Input: part model. Units: mm. Frame: model coordinates. A direction names the side the tool comes from. Coordinates: 2 decimals unless noted, no trailing zeros. Order: outer loops, then holes, each group sorted by start corner. A loop starts at its lowest first (then second) coordinate and runs counter-clockwise, first axis right, second up. Notation, with made-up numbers: (-27, -31) - (7, -31) arc R33 cw to (7, -3) - close; hole circle Ø5 at (3.25, 78.25). An arc over 180 degrees is marked (long way). One line per question, with ' | ' between items.
from build123d import *

# Parameters (mm, degrees)
SKETCH1_R           = 3
SKETCH1_R_2         = 2
BOSS_EXTRUDE1_DEPTH = 5


with BuildPart() as part:
    # Sketch1 → Boss-Extrude1 (new body)
    with BuildSketch(Plane(origin=(0, 0, 0), x_dir=(0, 0, -1), z_dir=(1, 0, 0))):
        Polygon((-32.401546808, -7.5), (3.598453192, -7.5), (6.598453192, -4.5), (24.598453192, -4.5), (27.598453192, -7.5), (63.598453192, -7.5), (54.938199155, 7.5), (51.938199155, 7.5), (45.876021328, 18), (51.938199155, 28.5), (54.938199155, 28.5), (63.598453192, 43.5), (27.598453192, 43.5), (24.598453192, 40.5), (6.598453192, 40.5), (3.598453192, 43.5), (-32.401546808, 43.5), (-23.74129277, 28.5), (-20.74129277, 28.5), (-14.679114943, 18), (-20.74129277, 7.5), (-23.74129277, 7.5), align=None)
        Circle(SKETCH1_R, mode=Mode.SUBTRACT)
        with Locations((38.848942605, 0)):
            Circle(SKETCH1_R, mode=Mode.SUBTRACT)
        with Locations((31.196906385, 36)):
            Circle(SKETCH1_R, mode=Mode.SUBTRACT)
        with Locations((-7.65203622, 36)):
            Circle(SKETCH1_R, mode=Mode.SUBTRACT)
        with Locations((15.598453192, 18)):
            Circle(SKETCH1_R_2, mode=Mode.SUBTRACT)
        with Locations((-2.401546808, 18)):
            Circle(SKETCH1_R_2, mode=Mode.SUBTRACT)
        with Locations((33.598453192, 18)):
            Circle(SKETCH1_R_2, mode=Mode.SUBTRACT)
    extrude(amount=BOSS_EXTRUDE1_DEPTH)


solid = part.part
Item 1: Section D-D on z = -22.5. Return the cut outline in (x, y).
Data:
outline: (0, -4.5) - (5, -4.5) - (5, 40.5) - (0, 40.5) - close
Item 2: Section C-C on z = -40. Return the cut outline in (x, y).
Data:
outline: (0, -7.5) - (5, -7.5) - (5, -2.77) - (0, -2.77) - close; (0, 2.77) - (5, 2.77) - (5, 43.5) - (0, 43.5) - close
Item 3: Ray query, line 1 (Y direction, x = 1.5, z = 0); line 2 (Z direction, x = 4.1, y = 35); line 3 (Z direction, x = 3.55, y = -5). Return the intervals inside material, ascending.
Data:
line 1: -7.5 to -3, 3 to 43.5 | line 2: -58.69 to -34.03, -28.37 to 4.82, 10.48 to 27.49 | line 3: -62.16 to -25.1, -6.1 to 30.96
Item 4: Section B-B on y = 0. Return the cut outline in (x, z).
Data:
outline: (0, -59.27) - (5, -59.27) - (5, -41.85) - (0, -41.85) - close; (0, -35.85) - (5, -35.85) - (5, -3) - (0, -3) - close; (0, 3) - (5, 3) - (5, 28.07) - (0, 28.07) - close
Item 5: Draft query along Z for faces 5 (the face through (2.46, 35.9, -59.21)), 6 (the face through (2, 28.5, -53)), 7 (the face through (2, 40.5, -16)). Return one class per face: released by +Z, released by -Z, zero draft, split by the parting line, or undercut.
Data:
face 5: released by -Z | face 6: zero draft | face 7: undercut
Item 6: Section A-A on x = 3.95. Count the separate pieces of the cut face and the enclosed holes in it, and give its area (3 significant figures).
Data:
separate pieces: 1 | enclosed holes: 7 | area: 3,740 mm^2
Item 7: Contact query for flat-ended pins moving along their axis: P1, Ø1.5, axis at x = 1.5, y = 16.5, coming from the +Z side; P2, Ø2.5, axis at x = 2, z = -19, coming from the +Y side. Output: stop coordinate, or through.
Data:
P1: z = 15.98 | P2: y = 40.5
Item 8: Access query for faces 1 (the face through (2, 7.5, 22)), 2 (the face through (2, 0, 3)), 3 (the face through (2, -4.5, -15)), 4 (the face through (2.465, 12.676, -48.95)). Directions: +Z, -Z, +X, -X, +Y, -Y. A direction counts if a zero-diameter tool reaches every point of the face in a straight line with its end or side. Return the directions, or none.
Data:
face 1: +Z, +X, -X | face 2: +X, -X | face 3: +X, -X, -Y | face 4: -Z, +X, -X
